Source: CAD feature listing. Evaluate the final solid. Frame: model axes, mm. A direction names the side the tool comes from. Give positions to 0.01 mm unless a question says otherwise; leave off trailing zeros. Order: outer loops, then holes, each group sorted by start corner. A loop starts at its lowest first (then second) coordinate and runs counter-clockwise, first axis right, second up. Notation, with made-up numbers: (-2.75, 84.5) - (10.25, 84.5) arc R29 cw to (10.25, 110.5) - close; hole circle Ø5 at (30, 33.25). An arc over 180 degrees is marked (long way). Use CSV: the item, a comma, the result in double quotes.
Autodesk Inventor part; units mm, degrees
ref_plane "YZ Plane" through (0, 0, 0) normal (1, 0, 0) x (0, 1, 0)
ref_plane "XZ Plane" through (0, 0, 0) normal (0, 1, 0) x (-1, 0, 0)
ref_plane "XY Plane" through (0, 0, 0) normal (0, 0, 1) x (1, 0, 0)
sketch "Sketch1" plane through (0, 0, 0) normal (0, 0, 1) x (1, 0, 0)
  line L0 (-160, 100) -> (160, 100)
  line L1 (160, 100) -> (160, -100)
  line L2 (160, -100) -> (-160, -100)
  line L3 (-160, -100) -> (-160, 100)
  point P0 (0, 0)
  dimension "d0" = 320
  dimension "d1" = 200
  dimension "d2" = 160
  dimension "d3" = 100
extrude "Extrusion1" add sketch "Sketch1" along normal blind 19.05
sketch "Sketch2" plane through (0, 0, 0) normal (0, 0, -1) x (-1, 0, 0)
  circle A0 centre (150, 90) radius 2.5
  circle A1 centre (85.4, 90.7874) radius 2.0701
  circle A2 centre (85.4, -89.2126) radius 2.5
  circle A3 centre (150, -90) radius 2.5
  circle A4 centre (10, 0) radius 2.067
  circle A5 centre (-10, 0) radius 2.067
  circle A6 centre (-85.4, -89.2126) radius 2.0701
  circle A7 centre (-150, -90) radius 2.5
  circle A8 centre (-85.4, 90.7874) radius 2.0701
  circle A9 centre (-150, 90) radius 2.5
  circle A10 centre (-150, -90) radius 5
  circle A11 centre (-85.4, -89.2126) radius 5
  circle A12 centre (-150, 90) radius 5
  circle A13 centre (-85.4, 90.7874) radius 6
  circle A14 centre (-10, 0) radius 5
  circle A15 centre (10, 0) radius 5
  circle A16 centre (85.4, 90.7874) radius 6
  circle A17 centre (150, 90) radius 5
  circle A18 centre (85.4, -89.2126) radius 6
  circle A19 centre (150, -90) radius 5
  point P0 (0, 0)
  dimension "d6" = 10
  dimension "d7" = 10
  dimension "d8" = 10
  dimension "d9" = 12
  dimension "d10" = 10
  dimension "d11" = 10
  dimension "d12" = 12
  dimension "d13" = 10
  dimension "d14" = 12
  dimension "d15" = 10
extrude "Extrusion2" cut sketch "Sketch2" against normal through all contours A0 | A1 | A2 | A3 | A4 | A5 | A6 | A7 | A8 | A9 | A10 | A11 | A12 | A13 | A14 | A15 | A16 | A17 | A18 | A19
sketch "Sketch5" plane through (0, 0, 19.05) normal (0, 0, 1) x (1, 0, 0)
  circle A0 centre (-120, 90) radius 2.75
  circle A1 centre (-120, -90) radius 2.75
  circle A2 centre (120, -90) radius 2.75
  circle A3 centre (120, 90) radius 2.75
  point P0 (0, 0)
hole "Hole1" at (-120, 90, 19.05) at (-120, -90, 19.05) at (120, -90, 19.05) at (120, 90, 19.05) direction (0, 0, -1) diameter 5 end through all counterbore diameter 10 counterbore depth 12
properties part number "wasteboard" material "Wood"
Item 1: Set-up query: faces 5 (the flat face through (-2, 100, 9)), 6 (the flat face through (122, -92, 7.05)). Return all of +Z, -Z, +X, -X, +Y, -Y with unobstructed straight access to the full face (end or side cutting, diameter ignored); none if empty.
Filled in:
face 5,"+Z, -Z, +X, -X, +Y"
face 6,"+Z"
Item 2: Section A-A on x = -150. Return the cut outline in (y, z).
Filled in:
outline,"(-100, 0) - (-95, 0) - (-95, 19.05) - (-100, 19.05) - close; (-85, 0) - (85, 0) - (85, 19.05) - (-85, 19.05) - close; (95, 0) - (100, 0) - (100, 19.05) - (95, 19.05) - close"
Item 3: Section C-C on x = 10. Return the cut outline in (y, z).
Filled in:
outline,"(-100, 0) - (-5, 0) - (-5, 19.05) - (-100, 19.05) - close; (5, 0) - (100, 0) - (100, 19.05) - (5, 19.05) - close"
Item 4: First-contact query: pin 1 (3 mm diameter, centred on x = 119, y = -92, fed in from +Z). Flat tip, straight axial feed; report the tip coordinate or a pass-through.
Filled in:
pin 1,"stops at z = 7.05"
Item 5: Section D-D on z = 13.25. Count the separate pieces of the cut face and the enclosed holes in it, then the cut area to 3 significant figures.
Filled in:
separate pieces,"1"
enclosed holes,"14"
area,"62,800 mm2"
Item 6: Mould query, pull axis X, two halves, no side actions, for faces 1 (the flat face through (-160, -1, 9)), 2 (the flat face through (-2, 1, 0)), 3 (the flat face through (-118, -92, 7.05)), 4 (the cylindrical face through (-118.085, 85.381, 12.966)). Classes: released by +X, released by -X, zero draft, split by the parting line, or undercut.
Filled in:
face 1,"released by -X"
face 2,"zero draft"
face 3,"undercut"
face 4,"undercut"
Item 7: Material intervals for line 1 (Y direction, x = -120, z = 5); line 2 (Y direction, x = -10, z = 6.75), sorted ascending. Write a range as from..to.
Filled in:
line 1,"y = -100..-92.5, -87.5..87.5, 92.5..100"
line 2,"y = -100..-5, 5..100"
Item 8: Section B-B on y = 0. Return the cut outline in (x, z), then the cut area to 4 significant figures.
Filled in:
outline,"(-160, 0) - (-15, 0) - (-15, 19.05) - (-160, 19.05) - close; (-5, 0) - (5, 0) - (5, 19.05) - (-5, 19.05) - close; (15, 0) - (160, 0) - (160, 19.05) - (15, 19.05) - close"
area,"5,715 mm2"
